Input: part model. Units: mm. Frame: model coordinates. Coordinates: 2 decimals unless noted, no trailing zeros. Order: outer loops, then holes, each group sorted by start corner. A loop starts at its lowest first (then second) coordinate and runs counter-clockwise, first axis right, second up. Notation, with made-up numbers: (70.25, 66) - (124.25, 66) arc R13 cw to (124.25, 72) - close; hole circle Ø5 at (87, -39.5). An arc over 180 degrees is marked (long way). Use a Markdown table: item, result. Add a question column.
from build123d import *

# Parameters (mm, degrees)
EXTRUDE_1_DEPTH = 25
FILLET_1_R      = 3


with BuildPart() as part:
    # Эскиз1 → Бобышка-Вытянуть1 (new body)
    with BuildSketch(Plane.XY):
        with BuildLine():
            Line((-12.5, 0), (-12.5, -25))
            Line((-12.5, -25), (12.5, -25))
            Line((12.5, -25), (12.5, 0))
            ThreePointArc((12.5, 0), (0, 12.5), (-12.5, 0))
        make_face()
    extrude(amount=EXTRUDE_1_DEPTH)

    # Скругление1
    fillet_1_edges = [part.edges().sort_by_distance(p)[0] for p in [
        (12.5, -12.5, 25),
        (0, 12.5, 25),
        (-12.5, -12.5, 25),
    ]]
    fillet(fillet_1_edges, radius=FILLET_1_R)


solid = part.part
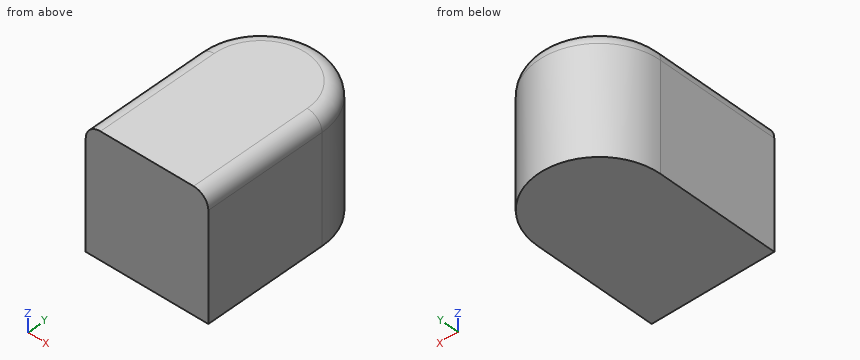
1) Contact query for flat-ended pins moving along their axis: P1, Ø4, axis at x = -4.5, z = 5.5, coming from the +Y side; P2, Ø6, axis at x = 6, z = 18.5, coming from the +Y side; P3, Ø1, axis at x = -5.5, y = 8.5, coming from the +Z side. Output: stop coordinate, or through.
2) Material intervals for L1, parallel to Y at x = 0.25, z = 3.5; L2, parallel to Z at x = 9.75, y = -21; L3, parallel to Y at x = 2.5, z = 9.5, sorted ascending.
3) Cut plane A-A (z = 6.5). Return the cut outline in (x, y).
Computed:
| question | item | result |
|---|---|---|
| 1 | P1 | stops at y = 12.25 |
| 1 | P2 | stops at y = 12.13 |
| 1 | P3 | stops at z = 25 |
| 2 | L1 | y = -25 to 12.5 |
| 2 | L2 | z = 0 to 24.99 |
| 2 | L3 | y = -25 to 12.25 |
| 3 | outline | (-12.5, -25) - (12.5, -25) - (12.5, 0) arc R12.5 ccw to (-12.5, 0) - close |
